Geometry: final body of the model. Coordinates: model frame, mm. A direction names the side the tool comes from. Coordinates: 2 decimals unless noted, no trailing zeros. Write each loop counter-clockwise with the first axis right and the second up, starting at its lowest first coordinate (ties: lowest second). Pieces come first, ordered by that corner, then holes. Notation, with made-up numbers: M 54.5,67.25 L 80.5,67.25 A18 cw 80.5,99.25 Z; hole C 3.5,46 d7. An arc over 180 degrees is marked long. Write item = value, one per line. Start each with the question number.
Item 1: Ray query, L1, parallel to Y at x = -38, z = 19; L2, parallel to X at y = -19, z = 25.75; L3, parallel to Y at x = -49.5, z = 16. Return the intervals inside material, ascending. Write a range as [from, to].
Item 2: Pull-direction query (X, two-part tool) for faces 1 (the flat face through (-47, -23.661, 24)), 2 (the flat face through (-48.971, 4.216, 18.697)), 3 (the flat face through (-32.94, 6.32, 23.6)); classes: +X half, -X half, draft (parallel to the pull), parting line (faces both ways), or undercut.
Item 3: Section B-B on y = -14. Output: boundary loops of the cut face in (x, z), plus the area to 3 significant figures.
Item 4: Section A-A on z = 25.25. Output: boundary loops of the cut face in (x, y), plus the area to 3 significant figures.
Item 5: Section D-D on z = 28.5. Output: boundary loops of the cut face in (x, y).
Item 6: Section C-C on x = -52.5. Output: boundary loops of the cut face in (y, z).
Item 7: Reachability of faces 4 (the flat face through (-35.13, 6.32, 27)), 5 (the flat face through (-48, 40.289, 22)), 6 (the flat face through (-57.9, 6.945, 29.916)), 7 (the flat face through (-57.842, 6.363, 27.092)), 8 (the flat face through (-49, 34.289, 17)) from +Z, -Z, +X, -X, +Y, -Y: full face, straight path, thin tool, end or side. Return the list, or none.
Item 8: First-contact query: pin 1 Ø2 at (x, y) = (-43.5, -1.5) entering from -Z; pin 2 Ø3 at (x, y) = (-53.5, 23.5) entering from -Z; pin 3 Ø1 at (x, y) = (-53, 5.5) entering from +Z. Flat tips, straight axial feed; report the tip coordinate or a pass-through.
from build123d import *

# Parameters (mm, degrees)
CROQUIS1_W              = 52
CROQUIS1_H              = 37
SALIENTE_EXTRUIR1_DEPTH = 3
REDONDEO1_R             = 3
CROQUIS2_R              = 1.5
CORTAR_EXTRUIR1_DEPTH   = 3
CROQUIS3_W              = 29
CROQUIS3_H              = 20
CROQUIS3_W_2            = 6
CROQUIS3_H_2            = 14
CORTAR_EXTRUIR2_DEPTH   = 3
SALIENTE_EXTRUIR2_DEPTH = 9
CROQUIS5_W              = 36
CROQUIS5_H              = 28.002550662
SALIENTE_EXTRUIR3_DEPTH = 10.3
CORTAR_EXTRUIR3_START   = -28.002551
CORTAR_EXTRUIR3_DEPTH   = 28.002551
SALIENTE_EXTRUIR4_DEPTH = 8.5
CROQUIS8_W              = 21.9
CROQUIS8_H              = 60.9
CORTAR_EXTRUIR4_DEPTH   = 5.5
CORTAR_EXTRUIR5_DEPTH   = 9
CORTAR_EXTRUIR6_START   = -28.002551
CROQUIS12_W             = 9
CROQUIS12_H             = 1.570892211
CORTAR_EXTRUIR6_DEPTH   = 28.002551
CROQUIS13_W             = 3
CROQUIS13_H             = 67
SALIENTE_EXTRUIR5_DEPTH = 12
CORTAR_EXTRUIR7_START   = -28.002551
CROQUIS14_W             = 31
CROQUIS14_H             = 9
CORTAR_EXTRUIR7_DEPTH   = 28.002551
CROQUIS17_R             = 1.5
SALIENTE_EXTRUIR6_DEPTH = 9
CORTAR_EXTRUIR8_START   = -37
CROQUIS18_W             = 54.197150846
CROQUIS18_H             = 9
CORTAR_EXTRUIR8_DEPTH   = 37
CROQUIS20_W             = 28
CROQUIS20_H             = 6
SALIENTE_EXTRUIR7_DEPTH = 3
CROQUIS21_W             = 20
CROQUIS21_H             = 4.5
CORTAR_EXTRUIR10_DEPTH  = 2
CROQUIS24_W             = 0.05
CROQUIS24_H             = 60.9
CORTAR_EXTRUIR13_DEPTH  = 5.5
CROQUIS25_W             = 64.228743672
CROQUIS25_H             = 61
CORTAR_EXTRUIR14_DEPTH  = 15
CROQUIS26_W             = 10.904109589
CROQUIS26_H             = 37
CORTAR_EXTRUIR15_DEPTH  = 15


with BuildPart() as part:
    # Croquis1 → Saliente-Extruir1 (new body)
    with BuildSketch(Plane.XY):
        with Locations((-39.296803653, 6.787671233)):
            Rectangle(CROQUIS1_W, CROQUIS1_H)
    extrude(amount=SALIENTE_EXTRUIR1_DEPTH)

    # Redondeo1
    redondeo1_edges = [part.edges().sort_by_distance(p)[0] for p in [
        (-65.296803653, 25.287671233, 1.5),
        (-65.296803653, -11.712328767, 1.5),
    ]]
    fillet(redondeo1_edges, radius=REDONDEO1_R)

    # Croquis2 → Cortar-Extruir1 (cut)
    with BuildSketch(Plane.XY.offset(3)):
        with Locations((-61.296803653, 21.287671233)):
            Circle(CROQUIS2_R)
        with Locations((-61.296803653, -7.712328767)):
            Circle(CROQUIS2_R)
        with Locations((-16.624072342, -7.712328767)):
            Circle(CROQUIS2_R)
        with Locations((-17.296803653, 21.287671233)):
            Circle(CROQUIS2_R)
    extrude(amount=-CORTAR_EXTRUIR1_DEPTH, mode=Mode.SUBTRACT)

    # Croquis3 → Cortar-Extruir2 (cut)
    with BuildSketch(Plane.XY.offset(3)):
        with Locations((-50.796803653, 6.787671233)):
            Rectangle(CROQUIS3_W, CROQUIS3_H)
        with Locations((-16.296803653, 6.787671233)):
            Rectangle(CROQUIS3_W_2, CROQUIS3_H_2)
    extrude(amount=-CORTAR_EXTRUIR2_DEPTH, mode=Mode.SUBTRACT)

    # Croquis4 → Saliente-Extruir2 (add)
    with BuildSketch(Plane.XY.offset(3)):
        Polygon((-57.296803653, 16.787671233), (-57.296803653, 20.790221895), (-26.296803653, 20.790221895), (-26.296803653, -7.212328767), (-57.296803653, -7.212328767), (-57.296803653, -3.212328767), (-36.296803653, -3.212328767), (-36.296803653, 16.787671233), align=None)
    extrude(amount=SALIENTE_EXTRUIR2_DEPTH)

    # Croquis5 → Saliente-Extruir3 (add)
    with BuildSketch(Plane.XY.offset(12)):
        with Locations((-44.296803653, 6.788946564)):
            Rectangle(CROQUIS5_W, CROQUIS5_H)
    extrude(amount=SALIENTE_EXTRUIR3_DEPTH)

    # Croquis6 → Cortar-Extruir3 (cut)
    with BuildSketch(Plane.XZ.offset(7.212328767).offset(CORTAR_EXTRUIR3_START)):
        Polygon((-35.296803653, 15), (-35.296803653, 12.995381041), (-26.296803653, 12.995381041), (-26.296803653, 14.757444162), (-26.296803653, 22.3), (-62.296803653, 22.3), align=None)
    extrude(amount=CORTAR_EXTRUIR3_DEPTH, mode=Mode.SUBTRACT)

    # Croquis7 → Saliente-Extruir4 (add)
    with BuildSketch(Plane(origin=(1.374852463, 0, 5.085070754), x_dir=(0.9653390502996949, 0, -0.2609990765625102), z_dir=(0.2609990765625102, 0, 0.9653390502996949))):
        Polygon((-65.957816682, 6.788946564), (-65.957816682, -26.711053436), (-37.957816682, -26.711053436), (-37.957816682, 40.288946564), (-65.957816682, 40.288946564), align=None)
    extrude(amount=SALIENTE_EXTRUIR4_DEPTH)

    # Croquis8 → Cortar-Extruir4 (cut)
    with BuildSketch(Plane(origin=(3.593344614, 0, 13.290452681), x_dir=(0.9653390502996949, 0, -0.26099907656251026), z_dir=(0.26099907656251026, 0, 0.9653390502996949))):
        with Locations((-51.957816682, 6.788946564)):
            Rectangle(CROQUIS8_W, CROQUIS8_H)
    extrude(amount=-CORTAR_EXTRUIR4_DEPTH, mode=Mode.SUBTRACT)

    # Croquis10 → Cortar-Extruir5 (cut)
    with BuildSketch(Plane(origin=(0, 20.790221895, 0), x_dir=(1, 0, 0), z_dir=(0, 1, 0))):
        Polygon((-62.296803653, -22.3), (-35.296803653, -15), (-35.296803653, -12), (-62.296803653, -19.3), align=None)
    extrude(amount=-CORTAR_EXTRUIR5_DEPTH, mode=Mode.SUBTRACT)

    # Croquis12 → Cortar-Extruir6 (cut)
    with BuildSketch(Plane(origin=(0, 20.790221895, 0), x_dir=(1, 0, 0), z_dir=(0, 1, 0)).offset(CORTAR_EXTRUIR6_START)):
        with Locations((-30.796803653, -12.209934936)):
            Rectangle(CROQUIS12_W, CROQUIS12_H)
    extrude(amount=CORTAR_EXTRUIR6_DEPTH, mode=Mode.SUBTRACT)

    # Croquis13 → Saliente-Extruir5 (add)
    with BuildSketch(Plane(origin=(3.593344614, 0, 13.290452681), x_dir=(0.9653390502996949, 0, -0.26099907656251026), z_dir=(0.26099907656251026, 0, 0.9653390502996949))):
        with Locations((-39.457816682, 6.788946564)):
            Rectangle(CROQUIS13_W, CROQUIS13_H)
    extrude(amount=SALIENTE_EXTRUIR5_DEPTH)

    # Croquis14 → Cortar-Extruir7 (cut)
    with BuildSketch(Plane.XZ.offset(7.212328767).offset(CORTAR_EXTRUIR7_START)):
        with Locations((-41.796803653, 7.5)):
            Rectangle(CROQUIS14_W, CROQUIS14_H)
    extrude(amount=CORTAR_EXTRUIR7_DEPTH, mode=Mode.SUBTRACT)


with BuildPart() as cortar_extruir7_piece_1:
    # of the separate pieces the step leaves, piece 1, a body of its own (cortar_extruir7_pieces)
    add(part.part.solids().sort_by_distance((-62.296803653, -26.711053436, 22.3))[0])



with BuildPart() as cortar_extruir7_piece_2:
    # of the separate pieces the step leaves, piece 2, a body of its own (cortar_extruir7_pieces)
    add(part.part.solids().sort_by_distance((-62.296803653, 25.287671233, 3))[0])


with BuildPart() as cortar_extruir7_piece_1_1:
    add(cortar_extruir7_piece_1.part)

    add(cortar_extruir7_piece_2.part)  # Saliente-Extruir6 merges Cortar-Extruir7 piece 2
    # Croquis17 → Saliente-Extruir6 (add)
    with BuildSketch(Plane.XY.offset(3)):
        with BuildLine():
            Line((-13.296803653, -0.212328767), (-19.296803653, -0.212328767))
            Line((-19.296803653, -0.212328767), (-19.296803653, 13.787671233))
            Line((-19.296803653, 13.787671233), (-13.296803653, 13.787671233))
            Line((-13.296803653, 13.787671233), (-13.296803653, 25.287671233))
            Line((-13.296803653, 25.287671233), (-62.296803653, 25.287671233))
            ThreePointArc((-62.296803653, 25.287671233), (-64.418123997, 24.408991576), (-65.296803653, 22.287671233))
            Line((-65.296803653, 22.287671233), (-65.296803653, 16.787671233))
            Line((-65.296803653, 16.787671233), (-36.296803653, 16.787671233))
            Line((-36.296803653, 16.787671233), (-36.296803653, -3.212328767))
            Line((-36.296803653, -3.212328767), (-65.296803653, -3.212328767))
            Line((-65.296803653, -3.212328767), (-65.296803653, -8.712328767))
            ThreePointArc((-65.296803653, -8.712328767), (-64.418123997, -10.833649111), (-62.296803653, -11.712328767))
            Line((-62.296803653, -11.712328767), (-13.296803653, -11.712328767))
            Line((-13.296803653, -11.712328767), (-13.296803653, -0.212328767))
        make_face()
        with Locations((-61.296803653, 21.287671233)):
            Circle(CROQUIS17_R, mode=Mode.SUBTRACT)
        with Locations((-61.296803653, -7.712328767)):
            Circle(CROQUIS17_R, mode=Mode.SUBTRACT)
        with Locations((-16.624072342, -7.712328767)):
            Circle(CROQUIS17_R, mode=Mode.SUBTRACT)
        with Locations((-17.296803653, 21.287671233)):
            Circle(CROQUIS17_R, mode=Mode.SUBTRACT)
    extrude(amount=SALIENTE_EXTRUIR6_DEPTH)

    # Croquis18 → Cortar-Extruir8 (cut)
    with BuildSketch(Plane.XZ.offset(11.712328767).offset(CORTAR_EXTRUIR8_START)):
        with Locations((-40.395379076, 4.5)):
            Rectangle(CROQUIS18_W, CROQUIS18_H)
    extrude(amount=CORTAR_EXTRUIR8_DEPTH, mode=Mode.SUBTRACT)

    # Croquis20 → Saliente-Extruir7 (add)
    with BuildSketch(Plane(origin=(1.374852463, 0, 5.085070754), x_dir=(-0.9653390502996949, 0, 0.26099907656251026), z_dir=(-0.26099907656251026, 0, -0.9653390502996949))):
        with Locations((51.957816682, 37.288946564)):
            Rectangle(CROQUIS20_W, CROQUIS20_H)
    extrude(amount=SALIENTE_EXTRUIR7_DEPTH)

    # Croquis21 → Cortar-Extruir10 (cut)
    with BuildSketch(Plane(origin=(0, 0, 9), x_dir=(-1, 0, 0), z_dir=(0, 0, -1))):
        with Locations((45.296803653, 19.037671233)):
            Rectangle(CROQUIS21_W, CROQUIS21_H)
        with Locations((45.296803653, -5.462328767)):
            Rectangle(CROQUIS21_W, CROQUIS21_H)
    extrude(amount=-CORTAR_EXTRUIR10_DEPTH, mode=Mode.SUBTRACT)

    # Croquis24 → Cortar-Extruir13 (cut)
    with BuildSketch(Plane(origin=(3.593344614, 0, 13.290452681), x_dir=(0.9653390502996949, 0, -0.26099907656251026), z_dir=(0.26099907656251026, 0, 0.9653390502996949))):
        with Locations((-40.982816682, 6.788946564)):
            Rectangle(CROQUIS24_W, CROQUIS24_H)
    extrude(amount=-CORTAR_EXTRUIR13_DEPTH, mode=Mode.SUBTRACT)

    # Croquis25 → Cortar-Extruir14 (cut)
    with BuildSketch(Plane(origin=(1.374852463, 0, 5.085070754), x_dir=(-0.9653390502996949, 0, 0.26099907656251026), z_dir=(-0.26099907656251026, 0, -0.9653390502996949))):
        with Locations((45.297379558, 3.788946564)):
            Rectangle(CROQUIS25_W, CROQUIS25_H)
    extrude(amount=CORTAR_EXTRUIR14_DEPTH, mode=Mode.SUBTRACT)


with BuildPart() as cortar_extruir14_piece_1:
    # of the separate pieces the step leaves, piece 1, a body of its own (cortar_extruir14_pieces)
    add(cortar_extruir7_piece_1_1.part.solids().sort_by_distance((-62.296803653, -26.711053436, 22.3))[0])


with BuildPart() as cortar_extruir14_piece_2:
    # of the separate pieces the step leaves, piece 2, a body of its own (cortar_extruir14_pieces)
    add(cortar_extruir7_piece_1_1.part.solids().sort_by_distance((-24.200913242, -11.712328767, 12))[0])

    # Croquis26 → Cortar-Extruir15 (cut)
    with BuildSketch(Plane.XY.offset(12)):
        with Locations((-18.748858448, 6.787671233)):
            Rectangle(CROQUIS26_W, CROQUIS26_H)
    extrude(amount=-CORTAR_EXTRUIR15_DEPTH, mode=Mode.SUBTRACT)


solid = cortar_extruir14_piece_1.part
Responses:
q1.L1 = [-26.71, -23.66], [37.24, 40.29]
q1.L2 = [-61.36, -58.2], [-35.47, -32.36]
q1.L3 = [34.29, 40.29]
q2.face_1 = undercut
q2.face_2 = -X half
q2.face_3 = +X half
q3.outline = M -62.3,22.3 L -35.27,14.99 L -29.92,34.78 L -32.81,35.56 L -37.38,18.67 L -58.57,24.4 L -57.13,29.71 L -60.08,30.51 Z
q3.area = 153 mm²
q4.outline = M -61.5,-26.71 L -40.64,-26.71 L -40.64,-23.66 L -58.34,-23.66 L -58.34,37.24 L -40.64,37.24 L -40.64,40.29 L -61.5,40.29 Z; M -35.6,-26.71 L -32.49,-26.71 L -32.49,40.29 L -35.6,40.29 Z
q4.area = 528 mm²
q5.outline = M -60.62,-26.71 L -52.66,-26.71 L -52.66,-23.66 L -57.46,-23.66 L -57.46,37.24 L -52.66,37.24 L -52.66,40.29 L -60.62,40.29 Z; M -34.72,-26.71 L -31.62,-26.71 L -31.62,40.29 L -34.72,40.29 Z
q6.outline = M -26.71,19.65 L 34.29,19.65 L 34.29,16.54 L 40.29,16.54 L 40.29,28.46 L 37.24,28.46 L 37.24,22.76 L -23.66,22.76 L -23.66,28.46 L -26.71,28.46 Z
q7.face_4 = +Z
q7.face_5 = +Z, -Z, +X, -X, +Y
q7.face_6 = +Z, +Y, -Y
q7.face_7 = none
q7.face_8 = -Z, -X, -Y
q8.pin_1 = 16.95
q8.pin_2 = 19.52
q8.pin_3 = 23.03
